from build123d import *

# Parameters (mm, degrees)
F0_W         = 116
F0_H         = 71
F0_R         = 1.75
F0_W_2       = 18
F0_H_2       = 8
F0_W_3       = 19
F0_H_3       = 10
F1_DEPTH     = 1.5
F2_W         = 116
F2_H         = 71
F2_W_2       = 112
F2_H_2       = 66
F3_DEPTH     = 10
F4_R         = 2.5
F5_R         = 1
F6_R         = 4.5
F6_R_2       = 2
F7_DEPTH     = 11
F8_T1_DEPTH  = 8
F8_T3_DEPTH  = 18
F8_T9_DEPTH  = 23.1433659759
F8_T13_DEPTH = 13.1433659759
F8_T20_DEPTH = 23.1433659759
F8_T24_DEPTH = 13.1433659759
F8_T31_DEPTH = 23.1433659759
F8_T35_DEPTH = 13.1433659759
F8_T42_DEPTH = 13.1433659759
F8_T46_DEPTH = 23.1433659759
F9_W         = 15.5
F9_H         = 9
F9_W_2       = 24
F9_H_2       = 5
F10_DEPTH    = 25
F11_DEPTH    = 25
F12_DEPTH    = 25


# Not quite as in the source:
# - a fillet or chamfer that OpenCascade refuses, or shapes differently, is made with other operations: its cross-section is extruded or revolved along the edge and cut away or added


with BuildPart() as f1:
    # F0 (on Top) → F1 (new body)
    with BuildSketch(Plane.XY):
        with Locations((58, 35.5)):
            Rectangle(F0_W, F0_H)
        with Locations((47.25, 26)):
            Circle(F0_R, mode=Mode.SUBTRACT)
        with Locations((58, 12)):
            Rectangle(F0_W_2, F0_H_2, mode=Mode.SUBTRACT)
        with Locations((68, 26)):
            Circle(F0_R, mode=Mode.SUBTRACT)
        with Locations((48, 51)):
            Circle(F0_R, mode=Mode.SUBTRACT)
        with Locations((30.5, 59)):
            Rectangle(F0_W_3, F0_H_3, mode=Mode.SUBTRACT)
        with Locations((68, 51)):
            Circle(F0_R, mode=Mode.SUBTRACT)
    extrude(amount=F1_DEPTH)

    # F2 (on face) → F3 (join)
    with BuildSketch(Plane.XY.offset(1.5)):
        with Locations((58, 35.5)):
            Rectangle(F2_W, F2_H)
        with Locations((58, 36)):
            Rectangle(F2_W_2, F2_H_2, mode=Mode.SUBTRACT)
    extrude(amount=F3_DEPTH)

    # F4
    f4_edges = [f1.edges().sort_by_distance(p)[0] for p in [
        (0, 0, 5.75),
        (116, 0, 5.75),
        (0, 71, 5.75),
        (116, 71, 5.75),
    ]]
    fillet(f4_edges, radius=F4_R)

    # F5
    f5_edges = [f1.edges().sort_by_distance(p)[0] for p in [
        (114, 3, 6.5),
        (2, 3, 6.5),
        (2, 69, 6.5),
        (114, 69, 6.5),
    ]]
    fillet(f5_edges, radius=F5_R)

    # F6 (on face) → F7 (join)
    with BuildSketch(Plane.XY.offset(1.5)):
        with Locations((7, 64)):
            Circle(F6_R)
        with Locations((7, 64)):
            Circle(F6_R_2, mode=Mode.SUBTRACT)
        with Locations((7, 8)):
            Circle(F6_R)
        with Locations((7, 8)):
            Circle(F6_R_2, mode=Mode.SUBTRACT)
        with Locations((109, 8)):
            Circle(F6_R)
        with Locations((109, 8)):
            Circle(F6_R_2, mode=Mode.SUBTRACT)
        with Locations((109, 64)):
            Circle(F6_R)
        with Locations((109, 64)):
            Circle(F6_R_2, mode=Mode.SUBTRACT)
    extrude(amount=F7_DEPTH)

    # F8: chamfer of 2 on 4 edges, made by hand

    # F8_s2 → F8_t1 (cut)
    with BuildSketch(Plane.XZ.offset(-16)):
        Polygon((69, 0), (67, 2), (67, 0), align=None)
        Polygon((47, 0), (49, 2), (49, 0), align=None)
    extrude(amount=F8_T1_DEPTH, mode=Mode.SUBTRACT)

    # F8_s4 → F8_t3 (cut)
    with BuildSketch(Plane.YZ.offset(49)):
        Polygon((6, 0), (8, 2), (8, 0), align=None)
        Polygon((18, 0), (16, 2), (16, 0), align=None)
    extrude(amount=F8_T3_DEPTH, mode=Mode.SUBTRACT)


with BuildPart() as f8_tool7:
    # F8_s8 → F8_t9 (new body)
    with BuildSketch(Plane.YZ.offset(49)):
        Polygon((18, 0), (16, 2), (16, 0), align=None)
    extrude(amount=F8_T9_DEPTH)

    split(bisect_by=Plane.YZ.offset(67), keep=Keep.TOP)


with BuildPart() as f8_tool11:
    # F8_s12 → F8_t13 (new body)
    with BuildSketch(Plane.XZ.offset(-21.1433659759)):
        Polygon((69, 0), (67, 2), (67, 0), align=None)
    extrude(amount=F8_T13_DEPTH)

    split(bisect_by=Plane.XZ.offset(-16), keep=Keep.BOTTOM)


with BuildPart() as f8_tool7_1:
    add(f8_tool7.part)

    # F8_t15: intersect F8_tool11
    add(f8_tool11.part, mode=Mode.INTERSECT)


with BuildPart() as f1_1:
    add(f1.part)

    # F8_t5: cut F8_tool7
    add(f8_tool7_1.part, mode=Mode.SUBTRACT)


with BuildPart() as f8_tool18:
    # F8_s19 → F8_t20 (new body)
    with BuildSketch(Plane.YZ.offset(72.1433659759)):
        Polygon((6, 0), (8, 2), (8, 0), align=None)
    extrude(amount=-F8_T20_DEPTH)

    split(bisect_by=Plane.YZ.offset(67), keep=Keep.TOP)


with BuildPart() as f8_tool22:
    # F8_s23 → F8_t24 (new body)
    with BuildSketch(Plane.XZ.offset(-16)):
        Polygon((69, 0), (67, 2), (67, 0), align=None)
    extrude(amount=F8_T24_DEPTH)

    split(bisect_by=Plane.XZ.offset(-8), keep=Keep.TOP)


with BuildPart() as f8_tool18_1:
    add(f8_tool18.part)

    # F8_t26: intersect F8_tool22
    add(f8_tool22.part, mode=Mode.INTERSECT)


with BuildPart() as f1_2:
    add(f1_1.part)

    # F8_t16: cut F8_tool18
    add(f8_tool18_1.part, mode=Mode.SUBTRACT)


with BuildPart() as f8_tool29:
    # F8_s30 → F8_t31 (new body)
    with BuildSketch(Plane.YZ.offset(67)):
        Polygon((6, 0), (8, 2), (8, 0), align=None)
    extrude(amount=-F8_T31_DEPTH)

    split(bisect_by=Plane.YZ.offset(49), keep=Keep.BOTTOM)


with BuildPart() as f8_tool33:
    # F8_s34 → F8_t35 (new body)
    with BuildSketch(Plane.XZ.offset(-2.8566340241)):
        Polygon((47, 0), (49, 2), (49, 0), align=None)
    extrude(amount=-F8_T35_DEPTH)

    split(bisect_by=Plane.XZ.offset(-8), keep=Keep.TOP)


with BuildPart() as f8_tool29_1:
    add(f8_tool29.part)

    # F8_t37: intersect F8_tool33
    add(f8_tool33.part, mode=Mode.INTERSECT)


with BuildPart() as f1_3:
    add(f1_2.part)

    # F8_t27: cut F8_tool29
    add(f8_tool29_1.part, mode=Mode.SUBTRACT)


with BuildPart() as f8_tool40:
    # F8_s41 → F8_t42 (new body)
    with BuildSketch(Plane.XZ.offset(-8)):
        Polygon((47, 0), (49, 2), (49, 0), align=None)
    extrude(amount=-F8_T42_DEPTH)

    split(bisect_by=Plane.XZ.offset(-16), keep=Keep.BOTTOM)


with BuildPart() as f8_tool44:
    # F8_s45 → F8_t46 (new body)
    with BuildSketch(Plane.YZ.offset(43.8566340241)):
        Polygon((18, 0), (16, 2), (16, 0), align=None)
    extrude(amount=F8_T46_DEPTH)

    split(bisect_by=Plane.YZ.offset(49), keep=Keep.BOTTOM)


with BuildPart() as f8_tool40_1:
    add(f8_tool40.part)

    # F8_t48: intersect F8_tool44
    add(f8_tool44.part, mode=Mode.INTERSECT)


with BuildPart() as f1_4:
    add(f1_3.part)

    # F8_t38: cut F8_tool40
    add(f8_tool40_1.part, mode=Mode.SUBTRACT)

    # F9 (on face) → F10 (cut)
    with BuildSketch(Plane(origin=(114, 0, 0), x_dir=(0, -1, 0), z_dir=(-1, 0, 0))):
        with Locations((-53.482233047, 11)):
            Rectangle(F9_W, F9_H)
        with Locations((-25.732233047, 13)):
            Rectangle(F9_W_2, F9_H_2)
    extrude(amount=-F10_DEPTH, mode=Mode.SUBTRACT)

    # F11 (cut): faces of the model
    f11_faces = [f1_4.faces().sort_by_distance(p)[0] for p in [
        (7, 8, 1.5),
        (7, 64, 1.5),
        (109, 8, 1.5),
        (109, 64, 1.5),
    ]]
    extrude(f11_faces, amount=-F11_DEPTH, mode=Mode.SUBTRACT)

    # F9 (on face) → F12 (cut)
    with BuildSketch(Plane(origin=(114, 0, 0), x_dir=(0, -1, 0), z_dir=(-1, 0, 0))):
        with Locations((-53.482233047, 11)):
            Rectangle(F9_W, F9_H)
        with Locations((-25.732233047, 13)):
            Rectangle(F9_W_2, F9_H_2)
    extrude(amount=F12_DEPTH, mode=Mode.SUBTRACT)


solid = f1_4.part
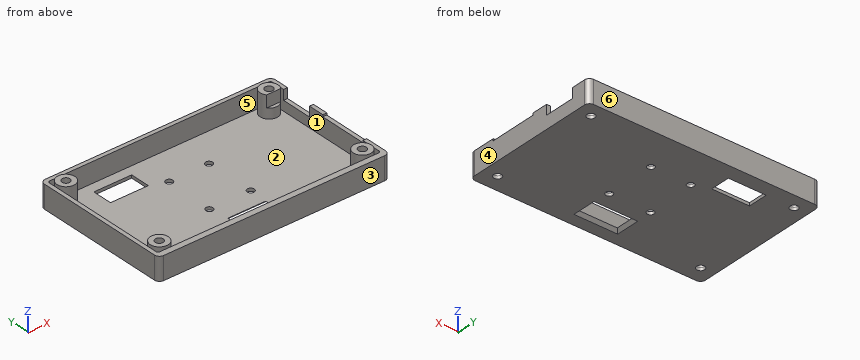
Could you check a few things on this model? Use its own coordinates, in mm. Face numbers are marked on the shaded views. A direction names the side the tool comes from. Coordinates: 2 decimals unless noted, no trailing zeros. Order: outer loops, then holes, each group sorted by start corner. A loop starts at its lowest first (then second) coordinate and runs counter-clockwise, first axis right, second up.
Q1. Suppose I cut it at B-B on x = 109. Please give me the cut outline in (y, z), and give its area (3 significant figures).
Q2. Thinking about a two-plate mould opening in Y: for the marked faces 1, 2, 3 and 4, which applies, released by +Y, released by -Y, zero draft, split by the parting line, or undercut?
Q3. Please list where these lines run through material, in increasing order: L1, parallel to Y at x = 109, z = 0.75; L2, parallel to Y at x = 25.5, z = 8.25; L3, parallel to X at y = 22.5, z = 2.5.
Q4. Which directions (+Z, -Z, +X, -X, +Y, -Y) give clear straight access to the entire face, cutting with the end or side of a thin tool? Please do the marked faces 5 and 6.
Q5. Suppose I cut it at D-D on x = 87.5. Please give me the cut outline in (y, z).
Q6. Suppose I cut it at C-C on y = 26. Please give me the cut outline in (x, z).
Q7. Will these pins go through, and if not, where does the flat tip stop? pin 1 (4.5 mm diameter, centred on x = 109, y = 8, fed in from +Z); pin 2 (0.5 mm diameter, centred on x = 108.5, y = 60.5, fed in from +Z); pin 3 (1.1 mm diameter, centred on x = 115, z = 11, fed in from -Y).
Q8. Suppose I cut it at A-A on z = 3.5. Give the number of separate pieces and of enclosed holes in the cut face, and give its area (3 significant figures).
Answer:
1. outline: (0, 0) - (6, 0) - (6, 12.5) - (3.5, 12.5) - (3.5, 1.5) - (3, 1.5) - (3, 11.5) - (0, 11.5) - close; (10, 0) - (62, 0) - (62, 12.5) - (61.23, 12.5) - (61.23, 6.5) - (59.5, 6.5) - (59.5, 1.5) - (12.5, 1.5) - (12.5, 12.5) - (10, 12.5) - close; (66, 0) - (71, 0) - (71, 11.5) - (69, 11.5) - (69, 1.5) - (68.5, 1.5) - (68.5, 12.5) - (66, 12.5) - close
1. area: 244 mm2
2. face 1: undercut
2. face 2: undercut
2. face 3: released by -Y
2. face 4: zero draft
3. L1: y = 0 to 6, 10 to 62, 66 to 71
3. L2: y = 0 to 3, 69 to 71
3. L3: x = 0 to 2, 114 to 116
4. face 5: +Z
4. face 6: +Z, -Z, +X, -X, +Y
5. outline: (0, 0) - (71, 0) - (71, 11.5) - (69, 11.5) - (69, 1.5) - (3, 1.5) - (3, 11.5) - (0, 11.5) - close
6. outline: (0, 0) - (45.5, 0) - (45.5, 1.5) - (2, 1.5) - (2, 11.5) - (0, 11.5) - close; (49, 0) - (66.25, 0) - (66.25, 1.5) - (49, 1.5) - close; (69.75, 0) - (116, 0) - (116, 10.5) - (114, 10.5) - (114, 1.5) - (69.75, 1.5) - close
7. pin 1: stops at z = 12.5
7. pin 2: stops at z = 6.5
7. pin 3: stops at y = 0.19
8. separate pieces: 5
8. enclosed holes: 5
8. area: 1,040 mm2
